Here's how the part is built. I have some questions about the finished solid (model axes, mm). Give positions to 0.01 mm unless a question says otherwise; leave off trailing zeros. Order: outer loops, then holes, each group sorted by start corner. A loop starts at its lowest first (then second) coordinate and runs counter-clockwise, first axis right, second up.
from build123d import *

# Parameters (mm, degrees)
BOSS_EXTRUDE1_DEPTH = 6
FILLET1_R           = 0.5
SKETCH4_R           = 6
BOSS_EXTRUDE2_DEPTH = 6
SKETCH3_R           = 2
SKETCH3_R_2         = 6
CUT_EXTRUDE1_DEPTH  = 353.232447151


with BuildPart() as part:
    # Sketch2 → Boss-Extrude1 (new body)
    with BuildSketch(Plane(origin=(0, 0, 0), x_dir=(0, 0, -1), z_dir=(1, 0, 0))):
        Polygon((0, 352), (0, 0), (-25, 25), (-25, 327), align=None)
    extrude(amount=BOSS_EXTRUDE1_DEPTH)

    # Fillet1
    fillet1_edges = [part.edges().sort_by_distance(p)[0] for p in [
        (3, 352, 0),
        (3, 0, 0),
    ]]
    fillet(fillet1_edges, radius=FILLET1_R)

    # Sketch4 → Boss-Extrude2 (add)
    with BuildSketch(Plane(origin=(6, 0, 0), x_dir=(0, 0, -1), z_dir=(1, 0, 0))):
        with Locations((-12, 340)):
            Circle(SKETCH4_R)
    extrude(amount=-BOSS_EXTRUDE2_DEPTH)

    # Sketch3 → Cut-Extrude1 (cut, through all)
    with BuildSketch(Plane(origin=(6, 0, 0), x_dir=(0, 0, -1), z_dir=(1, 0, 0))):
        with Locations((-12, 340)):
            Circle(SKETCH3_R)
        with Locations((-12, 12)):
            Circle(SKETCH3_R_2)
    extrude(amount=-CUT_EXTRUDE1_DEPTH, mode=Mode.SUBTRACT)


solid = part.part
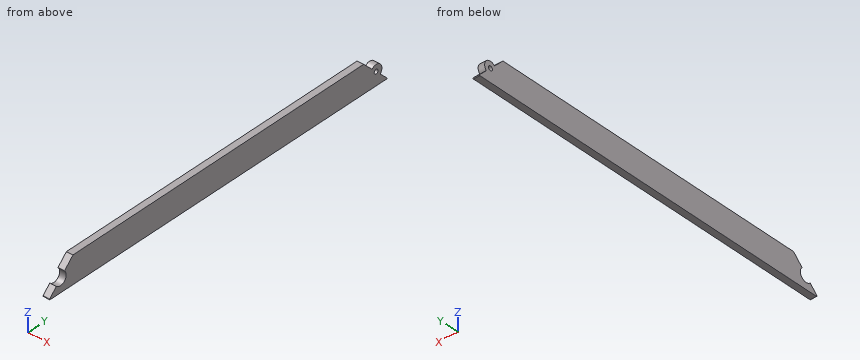
Q1. I need wall thicknesses on L1, parallel to Y at x = 1.4, z = 12; L2, parallel to Z at x = 3.4, y = 340; L3, parallel to Y at x = 5.4, z = 12.5. Which ranges of each line are inside material? Lowest first, please.
Filled sheet:
L1: y = 18 to 338, 342 to 346
L2: z = 0 to 10, 14 to 18
L3: y = 17.98 to 338.06, 341.94 to 345.98
Q2. If we section it at C-C on y = 12: List the corners of the cut face in (x, z) for me.
Filled sheet:
outline: (0, 0) - (6, 0) - (6, 6) - (0, 6) - close
Q3. I'm going to push flat-ended pins straight in: P1, Ø1, axis at x = 4.5, z = 10.5, coming from the +Y side; P2, Ø1.5, axis at x = 2, z = 18.5, coming from the -Y side. Where does each tip first touch, or does it pass through?
Filled sheet:
P1: stops at y = 345.92
P2: stops at y = 17.75
Q4. If we section it at A-A on x = 3.05: List the corners of the cut face in (y, z) for me.
Filled sheet:
outline: (0.85, 0.85) arc R0.5 ccw to (1.21, 0) - (350.79, 0) arc R0.5 ccw to (351.15, 0.85) - (344.24, 7.76) arc R6 ccw to (335.76, 16.24) - (327, 25) - (25, 25) - (16.24, 16.24) arc R6 cw to (7.76, 7.76) - close; hole circle Ø4 at (340, 12)
Q5. If we section it at B-B on z = 22: List the corners of the cut face in (x, y) for me, plus the area to 3 significant figures.
Filled sheet:
outline: (0, 22) - (6, 22) - (6, 330) - (0, 330) - close
area: 1,850 mm2
